Verification items for the finished model (mm, model axes). A direction names the side the tool comes from. Coordinates: 2 decimals unless noted, no trailing zeros. Loops run counter-clockwise (first coordinate to the right, second up) from the corner with the lowest first, then second, coordinate; pieces in that order, holes last. Notation, with made-up numbers: (1.25, -40) - (6.25, -40) arc R27 cw to (6.25, -8) - close; hole circle Ø8 at (87.25, 67.5). An arc over 180 degrees is marked (long way). One line per item, written item: value. Start each with the question number.
(1) Thickness scan on probe 1 along X at (y, z) = (7.75, -19); probe 2 along X at (y, z) = (23, -4); probe 3 along Z at (x, y) = (50, 4). Record the ranges inside material, lowest first. Write a range as [from, to].
(2) Section check B-B (z = 0). Record the boundary of the cut face in (x, y), plus the area to 3 significant figures.
(3) Draft check along X on faces 5 (the face through (38.5, 13.69, -29.38)), 6 (the face through (-71.943, 19.395, -21.9)), 7 (the face through (-1, 0, -16)). Enter one of: +X half, -X half, draft (parallel to the pull), parting line (faces both ways), or undercut.
(4) Section check A-A (y = 7). Record the boundary of the cut face in (x, z).
(5) Section check C-C (x = 47). Record the boundary of the cut face in (y, z).
(6) Gauge pin test, flat ends, axial feed: P1, Ø6, axis at y = 9.5, z = -3.5, coming from the +X side; P2, Ø7.5, axis at x = 9.5, y = 20, coming from the +Z side; P3, Ø8, axis at x = 52.5, z = 2.5, coming from the -Y side; P4, Ø9.5, axis at x = 50, z = -19, coming from the -Y side. Record the tip position at first contact, or that the pin passes through.
(7) Set-up check for faces 1 (the face through (0, 19, 5)), 2 (the face through (53, 16, -13)), 3 (the face through (1, 13, -29)), 4 (the face through (1, 6, -4)): record each of +Z, -Z, +X, -X, +Y, -Y from which the full face is reachable in a straight line by a thin tool's end or side.
(8) Section check D-D (z = 11.5). Record the boundary of the cut face in (x, y).
```python
from build123d import *
from build123d.topology import SkipClean

# Parameters (mm, degrees)
BOSS_EXTRU_1_DEPTH      = 27
ESQUISSE1_3_R           = 15
ENL_V_MAT_EXTRU_1_DEPTH = 12
TROU_TARAUD_M12X1_251_D = 10.8
PER_AGE1_D              = 12
PER_AGE1_DEPTH          = 27
PER_AGE1_CBORE_D        = 27
PER_AGE1_CBORE_DEPTH    = 11
PER_AGE1_TIP            = 3.605163714
CONG_1_R                = 6


with BuildPart() as part:
    # Esquisse1 → Boss.-Extru.1 (new body)
    with BuildSketch(Plane(origin=(0, 0, 0), x_dir=(1, 0, 0), z_dir=(0, 1, 0))):
        with BuildLine():
            Line((-74.347688243, -14.763645971), (-20, -5))
            Line((-20, -5), (20, -5))
            Line((20, -5), (74.347688243, -14.763645971))
            ThreePointArc((74.347688243, -14.763645971), (90.842168324, -5.778786733), (85.632401093, 12.26709629))
            Line((85.632401093, 12.26709629), (58.632401093, 31.26709629))
            ThreePointArc((58.632401093, 31.26709629), (48.294734794, 33.902753792), (38.819660113, 29))
            Line((38.819660113, 29), (-38.819660113, 29))
            ThreePointArc((-38.819660113, 29), (-48.294734794, 33.902753792), (-58.632401093, 31.26709629))
            Line((-58.632401093, 31.26709629), (-85.632401093, 12.26709629))
            ThreePointArc((-85.632401093, 12.26709629), (-90.842168324, -5.778786733), (-74.347688243, -14.763645971))
        make_face()
    extrude(amount=BOSS_EXTRU_1_DEPTH)

    # Esquisse1_3 → Enl_v. mat.-Extru.1 (cut)
    with SkipClean():  # keep this step's faces unmerged: merging them makes the solid invalid here
        with BuildSketch(Plane(origin=(0, 0, 0), x_dir=(1, 0, 0), z_dir=(0, 1, 0))):
            with BuildLine():
                Line((-74.347688243, -14.763645971), (-20, -5))
                Line((-20, -5), (0, -5))
                Line((0, -5), (20, -5))
                Line((20, -5), (74.347688243, -14.763645971))
                ThreePointArc((74.347688243, -14.763645971), (63.157831676, 5.778786733), (85.632401093, 12.26709629))
                Line((85.632401093, 12.26709629), (58.632401093, 31.26709629))
                ThreePointArc((58.632401093, 31.26709629), (63.31326437, 25.910643371), (65, 19))
                ThreePointArc((65, 19), (60.606601718, 8.393398282), (50, 4))
                Line((50, 4), (-50, 4))
                ThreePointArc((-50, 4), (-64.300462306, 14.472663274), (-58.632401093, 31.26709629))
                Line((-58.632401093, 31.26709629), (-85.632401093, 12.26709629))
                ThreePointArc((-85.632401093, 12.26709629), (-70.089356629, 13.31326437), (-62, 0))
                ThreePointArc((-62, 0), (-65.493813048, -9.623287475), (-74.347688243, -14.763645971))
            make_face()
            with Locations((77, 0)):
                Circle(ESQUISSE1_3_R)
            with Locations((-77, 0)):
                Circle(ESQUISSE1_3_R)
        extrude(amount=ENL_V_MAT_EXTRU_1_DEPTH, mode=Mode.SUBTRACT)

    # Trou taraud_ M12x1.251 (through all)
    with Locations(Plane(origin=(0, 12, 0), x_dir=(-1, 0, 0), z_dir=(0, -1, 0))):
        with Locations((-77, 0), (77, 0)):
            Hole(TROU_TARAUD_M12X1_251_D / 2)

    # Per_age1
    with Locations(Plane(origin=(0, 27, 0), x_dir=(1, 0, 0), z_dir=(0, 1, 0))):
        with Locations((-50, 19), (50, 19)):
            CounterBoreHole(PER_AGE1_D / 2, PER_AGE1_CBORE_D / 2, PER_AGE1_CBORE_DEPTH, depth=PER_AGE1_DEPTH)
            with Locations((0, 0, -(PER_AGE1_DEPTH + PER_AGE1_TIP / 2))):  # 118° drill point
                Cone(0, PER_AGE1_D / 2, PER_AGE1_TIP, mode=Mode.SUBTRACT)

    # Cong_1
    cong_1_edges = [part.edges().sort_by_distance(p)[0] for p in [
        (38.819660113, 13.5, -29),
        (-38.819660113, 13.5, -29),
    ]]
    fillet(cong_1_edges, radius=CONG_1_R)


solid = part.part
```
Responses:
1. probe 1: x = [-65, -56], [-44, 44], [56, 65]
1. probe 2: x = [-91.46, -80.63], [-73.37, 73.37], [80.63, 91.46]
1. probe 3: z = [-34, -25], [-13, -4]
2. outline: (-92, 12) - (-82.4, 12) - (-82.4, 27) - (-92, 27) - close; (-71.6, 12) - (71.6, 12) - (71.6, 27) - (-71.6, 27) - close; (82.4, 12) - (92, 12) - (92, 27) - (82.4, 27) - close
2. area: 2,440 mm²
3. face 5: undercut
3. face 6: -X half
3. face 7: draft
4. outline: (-50, -4) arc R15 ccw (long way) to (-40.28, -30.43) arc R6 cw to (-36.4, -29) - (36.4, -29) arc R6 cw to (40.28, -30.43) arc R15 ccw (long way) to (50, -4) - close; hole circle Ø12 at (-50, -19); hole circle Ø12 at (50, -19)
5. outline: (0, -33.7) - (27, -33.7) - (27, -32.16) - (16, -32.16) - (16, -24.2) - (0, -24.2) - close; (0, -13.8) - (16, -13.8) - (16, -5.84) - (27, -5.84) - (27, 9.85) - (12, 9.85) - (12, -4) - (0, -4) - close
6. P1: stops at x = 91.89
6. P2: stops at z = 5
6. P3: stops at y = 12
6. P4: passes through
7. face 1: +Z, +Y, -Y
7. face 2: +Y
7. face 3: -Z, +Y, -Y
7. face 4: +Z, +X, -X, -Y
8. outline: (-86.63, 12) - (-56.18, 12) - (-56.18, 27) - (-86.63, 27) - close; (56.18, 12) - (86.63, 12) - (86.63, 27) - (56.18, 27) - close
